Read the model definition and answer for the solid it produces. Units are mm, in the model's axes. A direction names the side the tool comes from. Round coordinates to 2 decimals unless told otherwise and drop trailing zeros. Write each loop counter-clockwise with the first axis right and the second up, starting at its lowest first coordinate (ties: lowest second). Pieces come first, ordered by that corner, then holes. Notation, with made-up numbers: (41, -6.75) - (61, -6.75) arc R16 ccw to (61, 3.25) - close; hole circle Ø11 at (8, -13.5). An arc over 180 degrees is marked (long way). Answer as CSV lines item,"result". Start each with the question number.
1) Consider line 1 along X through (y, z) = (19.55, 2.5); line 2 along Z through (x, y) = (-16, 21.3); line 3 along Y through (x, z) = (16, 2.5). Determine where each line is inside the solid, lowest interval first.
2) Find section A-A on y = 12.5. Determine the outline of the cut face in (x, z).
3) Which of the six approach directions +Z, -Z, +X, -X, +Y, -Y give full straight-line access (tool end or side, diameter ignored) to faces 1 (the cylindrical face through (-14.426, 19.965, 2.996)), 2 (the flat face through (-10, 22.5, 2))?
4) Find section B-B on y = 18.5. Determine the outline of the cut face in (x, z).
5) This flat-tipped pin is pushed along its axis until it touches: pin 1 (2.5 mm diameter, centred on x = -15, y = 12.5, fed in from -Z). Where does it stop, or does it pass through?
6) Find section C-C on z = 1.95. State how many separate pieces and enclosed holes the cut face has, then the cut area to 3 significant figures.
7) For a pull along X with two mould halves and no side action, classify faces 3 (the flat face through (0, -22.5, 2)), 4 (the conical face through (15.7, 16.7, 2.4)), 5 (the flat face through (20, 0, 2)) as +X half, -X half, draft (parallel to the pull), parting line (faces both ways), or undercut.
from build123d import *

# Parameters (mm, degrees)
F0_W     = 40
F0_H     = 45
F1_DEPTH = 5
F2_R     = 1.5
F3_DEPTH = 25
F5_DEPTH = 25
F7_D     = 3.3
F7_DEPTH = 5
F7_TIP   = 0.9914200214


with BuildPart() as f1:
    # F0 (on Top) → F1 (new body)
    with BuildSketch(Plane.XY):
        Rectangle(F0_W, F0_H)
    extrude(amount=F1_DEPTH)

    # F2 (on face) → F3 (cut)
    with BuildSketch(Plane.XY.offset(5)):
        with Locations((16, 12.5)):
            Circle(F2_R)
        with Locations((-15, 12.5)):
            Circle(F2_R)
    extrude(amount=-F3_DEPTH, mode=Mode.SUBTRACT)

    # F4 (on face) → F5 (cut)
    with BuildSketch(Plane.XY.offset(5)):
        Polygon((0.1732050808, 22.5), (-0.1732050808, 22.5), (0, 22.2), align=None)
    extrude(amount=-F5_DEPTH, mode=Mode.SUBTRACT)

    # F7
    with Locations(Plane(origin=(0, 22.5, 0), x_dir=(-1, 0, 0), z_dir=(0, 1, 0))):
        with Locations((-16, 2.5), (16, 2.5)):
            Hole(F7_D / 2, depth=F7_DEPTH)
            with Locations((0, 0, -(F7_DEPTH + F7_TIP / 2))):  # 118° drill point
                Cone(0, F7_D / 2, F7_TIP, mode=Mode.SUBTRACT)


solid = f1.part
Check values:
1,line 1,"x = -20 to -17.65, -14.35 to 14.35, 17.65 to 20"
1,line 2,"z = 0 to 0.85, 4.15 to 5"
1,line 3,"y = -22.5 to 11, 14 to 16.51"
2,outline,"(-20, 0) - (-16.5, 0) - (-16.5, 5) - (-20, 5) - close; (-13.5, 0) - (14.5, 0) - (14.5, 5) - (-13.5, 5) - close; (17.5, 0) - (20, 0) - (20, 5) - (17.5, 5) - close"
3,face 1,"+Y"
3,face 2,"+Z, -Z, +X, -X, +Y"
4,outline,"(-20, 0) - (20, 0) - (20, 5) - (-20, 5) - close; hole circle Ø3.3 at (-16, 2.5); hole circle Ø3.3 at (16, 2.5)"
5,pin 1,"passes through"
6,separate pieces,"1"
6,enclosed holes,"2"
6,area,"1,750 mm^2"
7,face 3,"draft"
7,face 4,"undercut"
7,face 5,"+X half"
